Print and shaded views of the part. All mm, measured from the part's lowest x, y and z. A direction names the side the tool comes from. Give positions to 0.01 mm unless a question says otherwise; leave off trailing zeros. Loops run counter-clockwise (first coordinate to the right, second up) from the corner with the lowest first, then second, coordinate; pieces in that order, holes last. Notation, with made-up numbers: (1.5, 43) - (28.5, 43) arc R13 cw to (28.5, 64) - close; hole circle Ø2 at (72.25, 15). An arc over 180 degrees is marked (long way). Return JSON: item names as keys, results as strings.
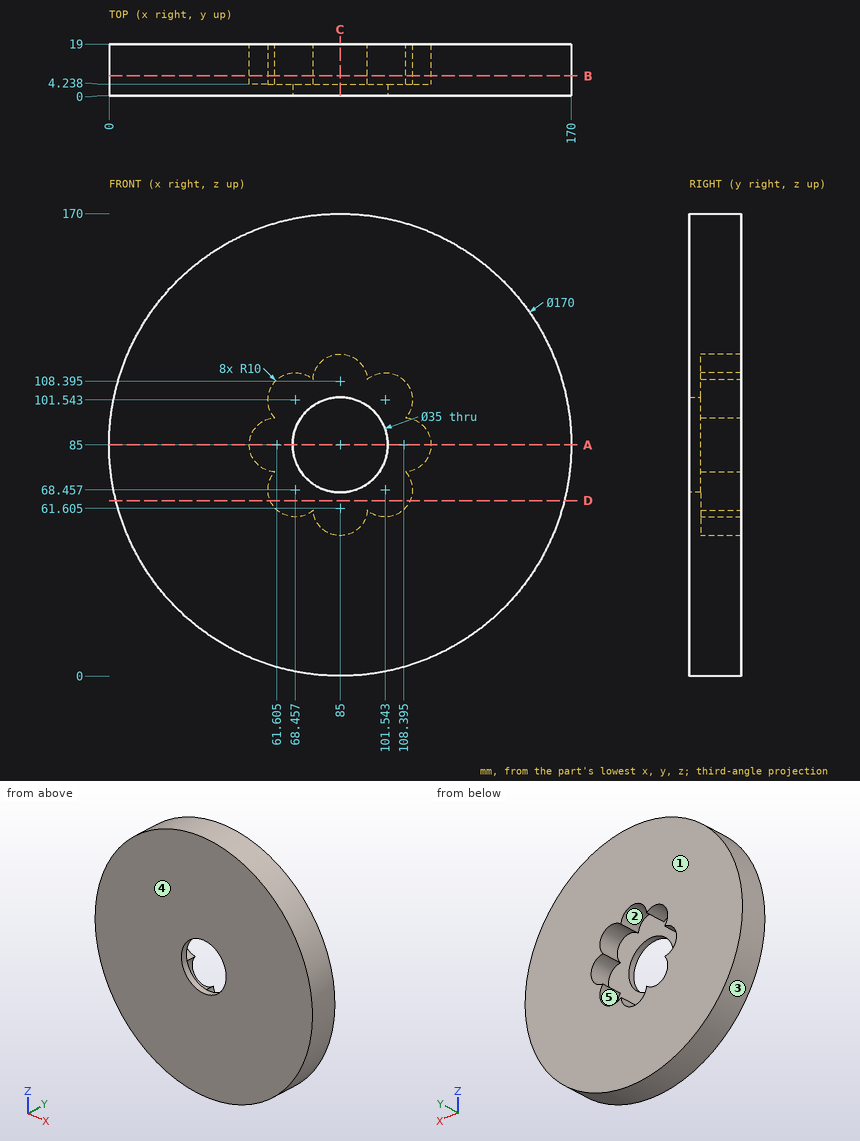
1. Cut at B-B, the plane y = 7.25. Write the cut outline in (x, z) (1 decimal).
Values follow:
{"outline": "circle Ø170 at (85, 85); hole (60.9, 75) arc R10 ccw to (75, 60.9) arc R10 ccw to (95, 60.9) arc R10 ccw to (109.1, 75) arc R10 ccw to (109.1, 95) arc R10 ccw to (95, 109.1) arc R10 ccw to (75, 109.1) arc R10 ccw to (60.9, 95) arc R10 ccw to start"}
2. Cut at A-A, the plane z = 85. Write the cut outline in (x, y) (1 decimal), plus the area to 3 significant figures.
Values follow:
{"outline": "(0, 0) - (67.5, 0) - (67.5, 4.2) - (51.6, 4.2) - (51.6, 19) - (0, 19) - close; (102.5, 0) - (170, 0) - (170, 19) - (118.4, 19) - (118.4, 4.2) - (102.5, 4.2) - close", "area": "2,100 mm²"}
3. Which spindle directions (+Z, -Z, +X, -X, +Y, -Y) get a long thin tool onto all of the face, cutting with end or side? Do the marked faces 4 and 5. Say none if no direction does.
Values follow:
{"face 4": "+Z, -Z, +X, -X, -Y", "face 5": "+Y"}
4. Drill centre lines: probe 1 along X at (y, z) = (2.7, 85); probe 2 along Y at (x, z) = (102, 90); probe 3 along Z at (x, y) = (61.5, 18) (1 decimal). Where is each one in solid material? Low to high.
Values follow:
{"probe 1": "x = 0 to 67.5, 102.5 to 170", "probe 2": "y = 0 to 4.24", "probe 3": "z = 3.3 to 61.3, 108.7 to 166.7"}
5. Cut at C-C, the plane x = 85. Write the cut outline in (y, z) (1 decimal), plus the area to 3 significant figures.
Values follow:
{"outline": "(0, 0) - (19, 0) - (19, 51.6) - (4.2, 51.6) - (4.2, 67.5) - (0, 67.5) - close; (0, 102.5) - (4.2, 102.5) - (4.2, 118.4) - (19, 118.4) - (19, 170) - (0, 170) - close", "area": "2,100 mm²"}
6. Pull direction Z, two halves, no side cores. Call the marked faces 1, 2 and 3: +Z half, -Z half, draft (parallel to the pull), parting line (faces both ways), or undercut.
Values follow:
{"face 1": "draft", "face 2": "undercut", "face 3": "parting line"}
7. Drop flat-ended pins along their axis: P1, Ø4, axis at y = 10, z = 18, coming from the +X side; P2, Ø3, axis at y = 9.5, z = 42.5, coming from the -X side; P3, Ø2, axis at x = 139.5, y = 14.5, coming from the +Z side. Give the stop position or say it passes through.
Values follow:
{"P1": "stops at x = 139.77", "P2": "stops at x = 10.54", "P3": "stops at z = 151.05"}
8. Cut at D-D, the plane z = 64.5. Write the cut outline in (x, y), plus the area to 4 significant figures.
Values follow:
{"outline": "(2.51, 0) - (167.49, 0) - (167.49, 19) - (110.73, 19) - (110.73, 4.24) - (59.27, 4.24) - (59.27, 19) - (2.51, 19) - close", "area": "2,375 mm²"}
